from build123d import *

# Parameters (mm, degrees)
SKETCH1_R           = 5
BOSS_EXTRUDE1_DEPTH = 3
CHAMFER1_SIZE       = 0.5
SKETCH2_R           = 3
BOSS_EXTRUDE2_DEPTH = 22
CHAMFER2_SIZE       = 0.5


with BuildPart() as part:
    # Sketch1 → Boss-Extrude1 (new body)
    with BuildSketch(Plane(origin=(0, 0, 0), x_dir=(-1, 0, 0), z_dir=(0, 1, 0))):
        with Locations(Location((0, 0, 0), (0, 0, 90))):
            Circle(SKETCH1_R)
    extrude(amount=BOSS_EXTRUDE1_DEPTH)

    # Chamfer1
    chamfer1_edges = [part.edges().sort_by_distance(p)[0] for p in [
        (0, 3, -5),
    ]]
    chamfer(chamfer1_edges, length=CHAMFER1_SIZE)

    # Sketch2 → Boss-Extrude2 (add)
    with BuildSketch(Plane.XZ):
        with Locations(Location((0, 0, 0), (0, 0, 270))):
            Circle(SKETCH2_R)
    extrude(amount=BOSS_EXTRUDE2_DEPTH)

    # Chamfer2
    chamfer2_edges = [part.edges().sort_by_distance(p)[0] for p in [
        (0, -22, 3),
    ]]
    chamfer(chamfer2_edges, length=CHAMFER2_SIZE)

    # Sketch3 → Cut-Revolve1 (revolve, cut)
    with BuildSketch(Plane.YZ):
        Polygon((-20.8, 3), (-20.8, 2.85), (-20, 2.85), (-20, 3), (-20, 3.35), (-20.8, 3.35), align=None)
    revolve(axis=Axis((0, 0, 0), (0, -1, 0)), mode=Mode.SUBTRACT)


solid = part.part
Could you check a few things on this model? Use its own coordinates, in mm. A direction names the side the tool comes from. Round coordinates to 2 decimals unless told otherwise and drop trailing zeros. Order: outer loops, then holes, each group sorted by start corner. A loop starts at its lowest first (then second) coordinate and runs counter-clockwise, first axis right, second up.
(1) Imagine slicing it at C-C (y = -10). Write out the boundary of the cut face in (x, z), plus the area to 3 significant figures.
Response values:
outline: circle Ø6 at (0, 0)
area: 28.3 mm2
(2) Which directions (+Z, -Z, +X, -X, +Y, -Y) give clear straight access to the entire face, cutting with the end or side of a thin tool? Please do faces 4 (the cylindrical face through (0.9, -9.86, -2.86)), 5 (the flat face through (0, -22, 0)).
Response values:
face 4: -Y
face 5: +Z, -Z, +X, -X, -Y
(3) If we mould it in two halves opening along Y, with no side actions, what happens to faces 1 (the flat face through (-3.3, 0, -0.1)), 2 (the cylindrical face through (-4.88, 1.23, -1.08)), 3 (the cylindrical face through (1.734, -20.394, -2.262))? For each: released by +Y, released by -Y, zero draft, split by the parting line, or undercut.
Response values:
face 1: released by -Y
face 2: zero draft
face 3: undercut
(4) Please list where these lines run through material, in increasing order: line 1 along Y through (x, z) = (0.25, -3.5); line 2 along Y through (x, z) = (2.75, -1); line 3 along X through (y, z) = (-11.5, 0.75).
Response values:
line 1: y = 0 to 3
line 2: y = -21.57 to -20.8, -20 to 3
line 3: x = -2.9 to 2.9
(5) Imagine slicing it at B-B (x = 0). Write out the boundary of the cut face in (y, z), plus the area to 3 significant figures.
Response values:
outline: (-22, -2.5) - (-21.5, -3) - (-20.8, -3) - (-20.8, -2.85) - (-20, -2.85) - (-20, -3) - (0, -3) - (0, -5) - (2.5, -5) - (3, -4.5) - (3, 4.5) - (2.5, 5) - (0, 5) - (0, 3) - (-20, 3) - (-20, 2.85) - (-20.8, 2.85) - (-20.8, 3) - (-21.5, 3) - (-22, 2.5) - close
area: 161 mm2
(6) I'm going to push flat-ended pins straight in: pin 1 (5 mm diameter, centred on y = -12, z = -3, fed in from +X); pin 2 (1 mm diameter, centred on x = -1.5, y = -7, fed in from +Z); pin 3 (3 mm diameter, centred on x = -0.5, z = -3.5, fed in from -Y); pin 4 (4 mm diameter, centred on y = -7.5, z = 0.5, fed in from -X). Where does each tip first touch, or does it pass through?
Response values:
pin 1: stops at x = 2.96
pin 2: stops at z = 2.83
pin 3: stops at y = -22
pin 4: stops at x = -3
(7) Imagine slicing it at A-A (z = 0). Write out the boundary of the cut face in (x, y).
Response values:
outline: (-5, 0) - (-3, 0) - (-3, -20) - (-2.85, -20) - (-2.85, -20.8) - (-3, -20.8) - (-3, -21.5) - (-2.5, -22) - (2.5, -22) - (3, -21.5) - (3, -20.8) - (2.85, -20.8) - (2.85, -20) - (3, -20) - (3, 0) - (5, 0) - (5, 2.5) - (4.5, 3) - (-4.5, 3) - (-5, 2.5) - close
